Verification items for the finished model (mm, model axes). Face numbers are marked on the shaded views. A direction names the side the tool comes from. Give positions to 0.01 mm unless a question says otherwise; leave off trailing zeros. Order: outer loops, then holes, each group sorted by start corner. A loop starts at its lowest first (then second) coordinate and runs counter-clockwise, first axis right, second up.
(1) Sectioned sample at C-C on z = -34.5. Record the cut outline in (x, y), plus the area to 3 significant figures.
(2) Access from +Z, -Z, +X, -X, +Y, -Y to the whole of each face (thin tool, end or side, straight path). Record for the marked faces 1, 2 and 3.
(3) Sectioned sample at A-A on y = -347. Record the cut outline in (x, z), plus the area to 3 significant figures.
(4) Gauge pin test, flat ends, axial feed: pin 1 (1.5 mm diameter, centred on x = -137.5, y = -1196, fed in from +Z); pin 2 (3 mm diameter, centred on y = -1415, z = -82.5, fed in from +X). Record the tip position at first contact, or that the pin passes through.
(5) Scan lines: L1, parallel to X at y = -1156, z = -195; L2, parallel to Z at x = -173, y = -483; L3, parallel to Y at x = 432, z = 264. Record each from-to range of solid material in increasing order.
(6) Sectioned sample at B-B on x = 418.5. Record the cut outline in (y, z), plus the area to 3 significant figures.
(7) Sectioned sample at D-D on z = 101. Record the cut outline in (x, y), plus the area to 3 significant figures.
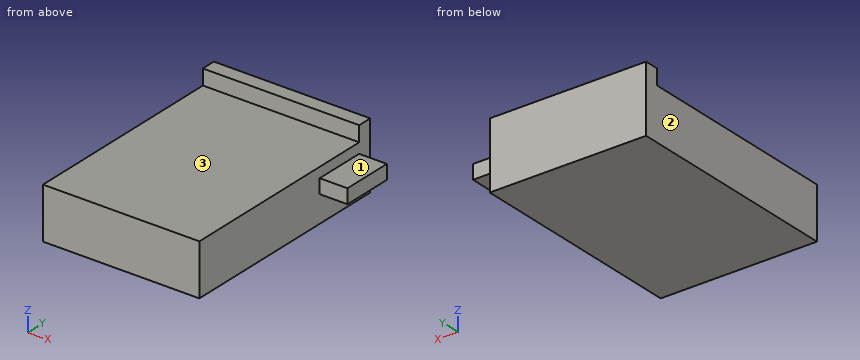
```python
from build123d import *

# Parameters (mm, degrees)
F0_W     = 1520
F0_H     = 500
F1_DEPTH = 2030
F2_W     = 1520
F2_H     = 650
F3_DEPTH = 140
F5_DEPTH = 270


with BuildPart() as f1:
    # F0 (on Front) → F1 (new body)
    with BuildSketch(Plane.XZ):
        Rectangle(F0_W, F0_H)
    extrude(amount=F1_DEPTH)



with BuildPart() as f3:
    # F2 (on face) → F3 (new body)
    with BuildSketch(Plane(origin=(0, 0, 0), x_dir=(-1, 0, 0), z_dir=(0, 1, 0))):
        with Locations((0, 75)):
            Rectangle(F2_W, F2_H)
    extrude(amount=F3_DEPTH)


with BuildPart() as f1_1:
    add(f1.part)

    add(f3.part)  # F5 merges F3
    # F4 (on face) → F5 (join)
    with BuildSketch(Plane.YZ.offset(760)):
        Polygon((0, 10), (-1.812994, 150), (-501.812994, 150), (-501.812994, 10), align=None)
    extrude(amount=F5_DEPTH)


solid = f1_1.part
```
Ans:
1. outline: (-760, -2030) - (760, -2030) - (760, 140) - (-760, 140) - close
1. area: 3,300,000 mm2
2. face 1: +Z, +X, +Y, -Y
2. face 2: +Z, -Z, -X, +Y, -Y
2. face 3: +Z, +X, -X, -Y
3. outline: (-760, -250) - (760, -250) - (760, 10) - (1030, 10) - (1030, 150) - (760, 150) - (760, 250) - (-760, 250) - close
3. area: 798,000 mm2
4. pin 1: stops at z = 250
4. pin 2: stops at x = 760
5. L1: x = -760 to 760
5. L2: z = -250 to 250
5. L3: y = 0 to 140
6. outline: (-2030, -250) - (140, -250) - (140, 400) - (0, 400) - (0, 250) - (-2030, 250) - close
6. area: 1,110,000 mm2
7. outline: (-760, -2030) - (760, -2030) - (760, -501.81) - (1030, -501.81) - (1030, -1.18) - (760, -1.18) - (760, 140) - (-760, 140) - close
7. area: 3,430,000 mm2
